```python
from build123d import *

# Parameters (mm, degrees)
SKETCH_W         = 40
SKETCH_H         = 87
PAD_DEPTH        = 5
SKETCH001_R      = 1.35
POCKET_DEPTH     = 10.001
SKETCH009_R      = 1.6
POCKET007_DEPTH  = 10.001
SKETCH010_W      = 5
SKETCH010_H      = 42
POCKET008_DEPTH  = 10.001
CHAMFER_SIZE     = 2
FILLET_R         = 1.5
CHAMFER001_SIZE2 = 20
CHAMFER001_SIZE  = 20
SKETCH011_W      = 22
SKETCH011_H      = 12
POCKET009_DEPTH  = 12
FILLET001_R      = 6
FILLET009_R      = 2
SKETCH012_W      = 27
SKETCH012_H      = 20
POCKET010_DEPTH  = 8
FILLET002_R      = 4
FILLET003_R      = 2
POCKET011_DEPTH  = 8
FILLET004_R      = 3
FILLET005_R      = 1.5
SKETCH014_R      = 1.35
POCKET012_DEPTH  = 10.001
SKETCH015_R      = 1.35
POCKET013_DEPTH  = 10.001
SKETCH016_W      = 34
SKETCH016_H      = 34
POCKET014_DEPTH  = 0.5
SKETCH017_R      = 1.35
POCKET015_DEPTH  = 13
FILLET010_R      = 1
FILLET011_R      = 1


with BuildPart() as part:
    # Sketch → Pad (new body, symmetric)
    with BuildSketch(Plane.XY):
        Rectangle(SKETCH_W, SKETCH_H)
    extrude(amount=PAD_DEPTH, both=True)

    # Sketch001 (on Face6 of Pad) → Pocket (cut, through all)
    with BuildSketch(Plane.XY.offset(5)):
        with Locations((17, -6.25)):
            Circle(SKETCH001_R)
        with Locations((-11, -6.25)):
            Circle(SKETCH001_R)
        with Locations((-17, -34.25)):
            Circle(SKETCH001_R)
    extrude(amount=-POCKET_DEPTH, mode=Mode.SUBTRACT)

    # Sketch009 (on Face5 of Pocket) → Pocket007 (cut, through all)
    with BuildSketch(Plane.XY.offset(5)):
        with Locations((-16, 3.5)):
            Circle(SKETCH009_R)
        with Locations((-3, 3.5)):
            Circle(SKETCH009_R)
        with Locations((10, 3.5)):
            Circle(SKETCH009_R)
    extrude(amount=-POCKET007_DEPTH, mode=Mode.SUBTRACT)

    # Sketch010 (on Face5 of Pocket007) → Pocket008 (cut, through all)
    with BuildSketch(Plane.XY.offset(5)):
        with Locations((17.5, 22.5)):
            Rectangle(SKETCH010_W, SKETCH010_H)
    extrude(amount=-POCKET008_DEPTH, mode=Mode.SUBTRACT)

    # Chamfer
    chamfer_edges = [part.edges().sort_by_distance(p)[0] for p in [
        (8.4, 3.5, 5),
        (-4.6, 3.5, 5),
        (-17.6, 3.5, 5),
    ]]
    chamfer(chamfer_edges, length=CHAMFER_SIZE)

    # Fillet
    fillet_edges = [part.edges().sort_by_distance(p)[0] for p in [
        (20, 1.5, 0),
        (15, 1.5, 0),
    ]]
    fillet(fillet_edges, radius=FILLET_R)

    # Chamfer001
    chamfer001_edges = [part.edges().sort_by_distance(p)[0] for p in [
        (-20, 43.5, 0),
    ]]
    chamfer001_side = part.faces().sort_by_distance((-2.5, 43.5, 0))[0]
    chamfer(chamfer001_edges, length=CHAMFER001_SIZE, length2=CHAMFER001_SIZE2, reference=chamfer001_side)

    # Sketch011 (on Face1 of Chamfer001) → Pocket009 (cut)
    with BuildSketch(Plane.XY.offset(5)):
        with Locations((3.5, -9.5)):
            Rectangle(SKETCH011_W, SKETCH011_H)
    extrude(amount=-POCKET009_DEPTH, mode=Mode.SUBTRACT)

    # Fillet001
    fillet001_edges = [part.edges().sort_by_distance(p)[0] for p in [
        (-7.5, -3.5, 0),
        (14.5, -15.5, 0),
    ]]
    fillet(fillet001_edges, radius=FILLET001_R)

    # Fillet009
    fillet009_edges = [part.edges().sort_by_distance(p)[0] for p in [
        (14.5, -3.5, 0),
        (-7.5, -15.5, 0),
    ]]
    fillet(fillet009_edges, radius=FILLET009_R)

    # Sketch012 (on Face1 of Fillet001) → Pocket010 (cut)
    with BuildSketch(Plane.XY.offset(5)):
        with Locations((1.5, -28.5)):
            Rectangle(SKETCH012_W, SKETCH012_H)
    extrude(amount=-POCKET010_DEPTH, mode=Mode.SUBTRACT)

    # Fillet002
    fillet002_edges = [part.edges().sort_by_distance(p)[0] for p in [
        (-12, -18.5, 1),
        (-12, -38.5, 1),
        (15, -38.5, 1),
        (15, -18.5, 1),
    ]]
    fillet(fillet002_edges, radius=FILLET002_R)

    # Fillet003
    fillet003_edges = [part.edges().sort_by_distance(p)[0] for p in [
        (-12, -28.5, -3),
    ]]
    fillet(fillet003_edges, radius=FILLET003_R)

    # Sketch013 (on Face4 of Fillet003) → Pocket011 (cut)
    with BuildSketch(Plane.XY.offset(5)):
        Polygon((-15, 21.428932), (1.071068, 37.5), (8, 37.5), (8, 15.428932), (-15, 15.428932), align=None)
    extrude(amount=-POCKET011_DEPTH, mode=Mode.SUBTRACT)

    # Fillet004
    fillet004_edges = [part.edges().sort_by_distance(p)[0] for p in [
        (-15, 15.428932, 1),
        (-15, 21.428932, 1),
        (8, 15.428932, 1),
        (8, 37.5, 1),
        (1.071068, 37.5, 1),
    ]]
    fillet(fillet004_edges, radius=FILLET004_R)

    # Fillet005
    fillet005_edges = [part.edges().sort_by_distance(p)[0] for p in [
        (-3.5, 15.428932, -3),
    ]]
    fillet(fillet005_edges, radius=FILLET005_R)

    # Sketch014 (on Face4 of Fillet005) → Pocket012 (cut, through all)
    with BuildSketch(Plane.XY.offset(5)):
        with Locations((-15, 11.5)):
            Circle(SKETCH014_R)
        with Locations((5, 11.5)):
            Circle(SKETCH014_R)
    extrude(amount=-POCKET012_DEPTH, mode=Mode.SUBTRACT)

    # Sketch015 (on Face56 of Pocket012) → Pocket013 (cut, through all)
    with BuildSketch(Plane(origin=(0, 0, -5), x_dir=(1, 0, 0), z_dir=(0, 0, -1))):
        with Locations((12, 40.5)):
            Circle(SKETCH015_R)
    extrude(amount=-POCKET013_DEPTH, mode=Mode.SUBTRACT)

    # Sketch016 (on Face4 of Pocket013) → Pocket014 (cut)
    with BuildSketch(Plane.XY.offset(5)):
        with Locations((3, -26.5)):
            Rectangle(SKETCH016_W, SKETCH016_H)
    extrude(amount=-POCKET014_DEPTH, mode=Mode.SUBTRACT)

    # Sketch017 (on Face15 of Pocket014) → Pocket015 (cut)
    with BuildSketch(Plane.YZ.offset(20)):
        with Locations((13.5, 0)):
            Circle(SKETCH017_R)
        with Locations((26.5, 0)):
            Circle(SKETCH017_R)
        with Locations((39.5, 0)):
            Circle(SKETCH017_R)
    extrude(amount=-POCKET015_DEPTH, mode=Mode.SUBTRACT)

    # Fillet010
    fillet010_edges = [part.edges().sort_by_distance(p)[0] for p in [
        (-20, -43.5, 0),
        (-20, 23.5, 0),
        (0, 43.5, 0),
        (15, 43.5, 0),
        (20, -43.5, -0.25),
    ]]
    fillet(fillet010_edges, radius=FILLET010_R)

    # Fillet011
    fillet011_edges = [part.edges().sort_by_distance(p)[0] for p in [
        (20, -9.5, 4.75),
        (14.5, -9.5, 4.75),
        (-7.5, -9.5, 4.75),
        (-14, -9.5, 4.75),
        (-14, -43.5, 4.75),
    ]]
    fillet(fillet011_edges, radius=FILLET011_R)


solid = part.part
```
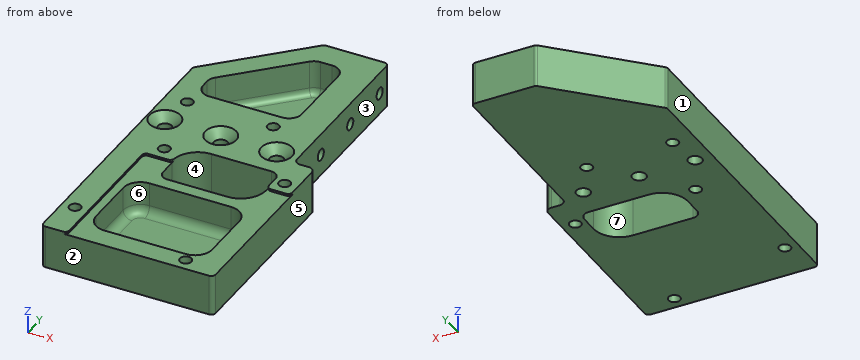
Geometry check sheet. Reference: the model listing, model coordinates, mm. Face numbers are marked on the shaded views. A direction names the side the tool comes from. Coordinates: 2 decimals unless noted, no trailing zeros. Order: outer loops, then holes, each group sorted by start corner. A loop starts at its lowest first (then second) coordinate and runs counter-clockwise, first axis right, second up. Notation, with made-up numbers: M -37,49.5 L 19,49.5 A30 ccw 19,88.5 Z; hole C -4,-29.5 d6. An arc over 180 degrees is marked long. Answer as a JSON object with one key per item and string values.
Q1. Release check for a two-part mould opening along X. For the marked faces 1, 2, 3 and 4 record: released by +X, released by -X, zero draft, split by the parting line, or undercut.
Results are:
{"face 1": "released by -X", "face 2": "zero draft", "face 3": "released by +X", "face 4": "undercut"}
Q2. Scan lines: line 1 (Y direction, x = 5, z = 4.25); line 2 (Y direction, x = 10, z = -2.5); line 3 (Y direction, x = -1.5, z = 4.75). Record each from-to range of solid material in increasing order.
Results are:
{"line 1": "y = -43.5 to -38.5, -18.5 to -15.5, -3.5 to 10.15, 12.85 to 15.43, 37.5 to 43.5", "line 2": "y = -43.5 to -37.82, -19.18 to -15.31, -3.5 to 1.9, 5.1 to 43.5", "line 3": "y = -3.5 to 0.5, 6.5 to 15.43, 34.93 to 42"}
Q3. Tool access check on the marked faces 5, 6 and 7. Record the directions out of +Z, -Z, +X, -X, +Y, -Y that give a thin tool (end or side, any length) a straight path to the whole face; none if there is none.
Results are:
{"face 5": "+Z, -Z, +X, +Y, -Y", "face 6": "+Z", "face 7": "+Z, -Z"}
Q4. Depth check by flat-ended pin: pin 1 Ø1.5 at (y, z) = (34, 3.5) entering from +X; pin 2 Ø8 at (x, y) = (4.5, -19) entering from +Z; pin 3 Ø13 at (x, y) = (6, -29.5) entering from +Z. Enter the tip coordinate at first touch or a pass-through.
Results are:
{"pin 1": "stops at x = 15", "pin 2": "stops at z = 4.5", "pin 3": "stops at z = -3"}
Q5. Cross-section at A-A on y = 39.5. Record the cut outline in (x, z), and give its area (3 significant figures).
Results are:
{"outline": "M -4,-5 L 15,-5 L 15,-1.35 L 7,-1.35 L 7,1.35 L 15,1.35 L 15,5 L -4,5 Z", "area": "168 mm²"}
